from build123d import *

# Parameters (mm, degrees)
SKETCH1_R               = 8.95
SKETCH1_W               = 9.9
SKETCH1_H               = 9.9
BOSS_EXTRUDE1_DEPTH     = 12
CUT_EXTRUDE2_DEPTH      = 18.441473562
CUT_EXTRUDE2_DEPTH_BACK = 18.441473562
SKETCH4_R               = 1.5


with BuildPart() as part:
    # Sketch1 → Boss-Extrude1 (new body)
    with BuildSketch(Plane(origin=(0, 0, 0), x_dir=(1, 0, 0), z_dir=(0, 1, 0))):
        with Locations(Location((0, 0, 0), (0, 0, 270))):
            Circle(SKETCH1_R)
        Rectangle(SKETCH1_W, SKETCH1_H, mode=Mode.SUBTRACT)
    extrude(amount=BOSS_EXTRUDE1_DEPTH)

    # Sketch4 → Cut-Extrude2 (cut, two sides: drawn at the far end of the back side and taken through both)
    with BuildSketch(Plane.XY.offset(-CUT_EXTRUDE2_DEPTH_BACK)):
        with Locations((0, 4.916404418)):
            Circle(SKETCH4_R)
    extrude(amount=CUT_EXTRUDE2_DEPTH + CUT_EXTRUDE2_DEPTH_BACK, mode=Mode.SUBTRACT)


solid = part.part
Build history of the part. All positions in model axes, mm. A direction names the side the tool comes from. Give positions to 0.01 mm unless a question says otherwise; leave off trailing zeros. Order: outer loops, then holes, each group sorted by start corner. A loop starts at its lowest first (then second) coordinate and runs counter-clockwise, first axis right, second up. Notation, with made-up numbers: M 67,22 L 122,22 A21 ccw 122,40 Z; hole C 9,65 d8. An arc over 180 degrees is marked long. Put each result on its own line as item: value.
Item 1: Slice it at A-A, the plane x = 0. Write the cut outline in (y, z).
From the geometry:
outline: M 0,-8.95 L 3.42,-8.95 L 3.42,-4.95 L 0,-4.95 Z; M 0,4.95 L 3.42,4.95 L 3.42,8.95 L 0,8.95 Z; M 6.42,-8.95 L 12,-8.95 L 12,-4.95 L 6.42,-4.95 Z; M 6.42,4.95 L 12,4.95 L 12,8.95 L 6.42,8.95 Z
Item 2: Slice it at D-D, the plane x = -4. Write the cut outline in (y, z), plus the area to 3 significant figures.
From the geometry:
outline: M 0,-8.01 L 12,-8.01 L 12,-4.95 L 0,-4.95 Z; M 0,4.95 L 12,4.95 L 12,8.01 L 0,8.01 Z
area: 73.4 mm2
Item 3: Slice it at B-B, the plane z = 0. Write the cut outline in (x, y).
From the geometry:
outline: M -8.95,0 L -4.95,0 L -4.95,12 L -8.95,12 Z; M 4.95,0 L 8.95,0 L 8.95,12 L 4.95,12 Z
Item 4: Probe line 1 (Y direction, x = 0, z = -5.9); line 2 (X direction, y = 4, z = -0.5); line 3 (Y direction, x = 1.25, z = -6.75). List the from-to ranges inside material, lowest first. Write a range as [from, to].
From the geometry:
line 1: y = [0, 3.42], [6.42, 12]
line 2: x = [-8.94, -4.95], [4.95, 8.94]
line 3: y = [0, 4.09], [5.75, 12]
Item 5: Flat gauge pins, fed straight in: pin 1 Ø3 at (y, z) = (4, 2) entering from -X; pin 2 Ø6 at (x, y) = (5, 6) entering from +Z; pin 3 Ø3 at (x, y) = (-5.5, 10) entering from +Z. Where does each tip first touch, or does it go through?
From the geometry:
pin 1: stops at x = -8.94
pin 2: stops at z = 8.72
pin 3: stops at z = 8.01
Item 6: Slice it at C-C, the plane y = 9.5. Write the cut outline in (x, z), plus the area to 3 significant figures.
From the geometry:
outline: C 0,0 d17.9; hole M -4.95,-4.95 L 4.95,-4.95 L 4.95,4.95 L -4.95,4.95 Z
area: 154 mm2
Item 7: Two-plate mould, pull along X, no slides. Class faces 3 (the flat face through (0, 7, 4.95)), 4 (the cylindrical face through (2.688, 5.916, 8.537)), 5 (the flat face through (-6, 0, 0)): +X half, -X half, draft (parallel to the pull), parting line (faces both ways), or undercut.
From the geometry:
face 3: undercut
face 4: parting line
face 5: draft
Item 8: 3-axis set-ups, long thin cutter, end or side, ignore diameter. For faces 1 (the flat face through (4.95, 6, 0)), 2 (the cylindrical face through (-0.195, 6.404, -6.98)): which of +Z, -Z, +X, -X, +Y, -Y reach the whole face in a straight line?
From the geometry:
face 1: +Y, -Y
face 2: +Z, -Z
